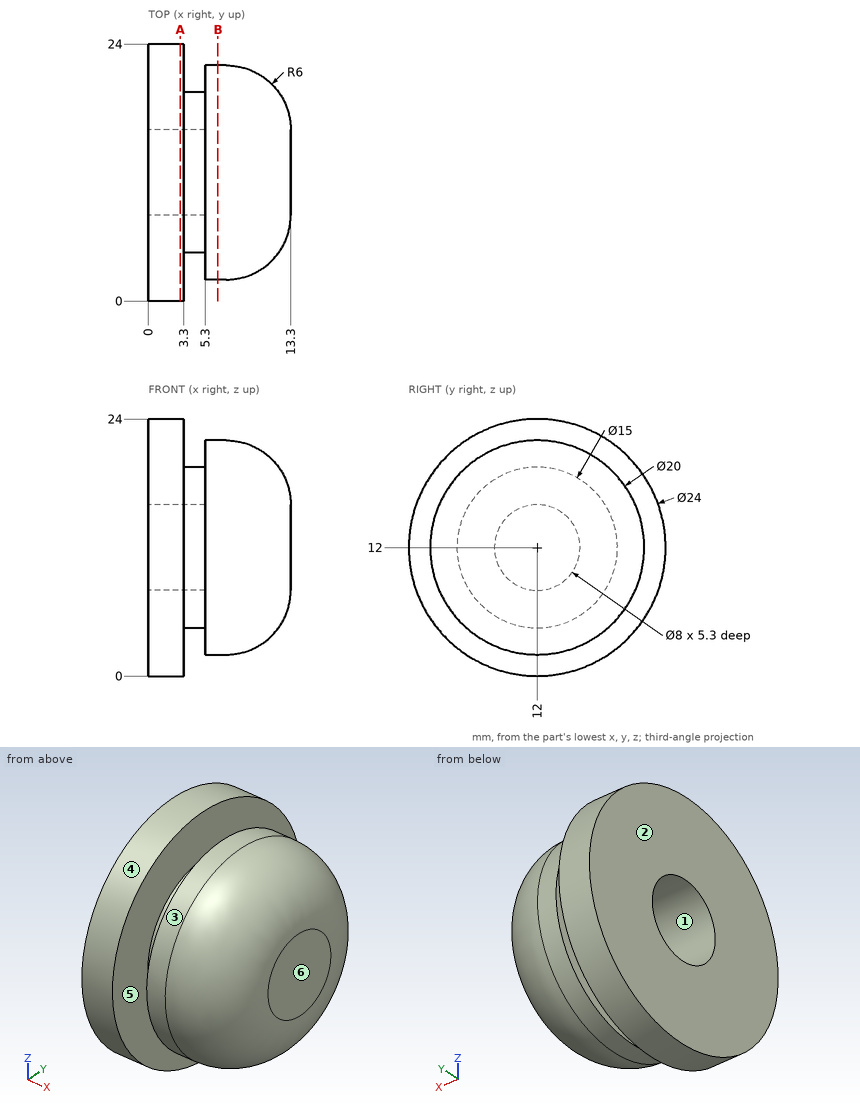
Geometry check sheet. Reference: drawing and pictorial views, mm from the part's lowest x, y, z. A direction names the side the tool comes from. Coordinates: 2 decimals unless noted, no trailing zeros. Loops run counter-clockwise (first coordinate to the right, second up) from the corner with the lowest first, then second, coordinate; pieces in that order, holes last. Notation, with made-up numbers: (20.5, -12.75) -> (46.5, -12.75) arc R24 ccw to (46.5, 25.25) -> close; hole circle Ø4 at (-18, 70.5). An arc over 180 degrees is marked (long way). Put each result on its own line as item: value.
1) Cross-section at B-B on x = 6.5. Record the boundary of the cut face in (y, z), plus the area to 3 significant figures.
Result set:
outline: circle Ø20 at (12, 12)
area: 314 mm^2
2) Tool access check on the marked faces 1, 2 and 3. Record the directions out of +Z, -Z, +X, -X, +Y, -Y that give a thin tool (end or side, any length) a straight path to the whole face; none if there is none.
Result set:
face 1: -X
face 2: +Z, -Z, -X, +Y, -Y
face 3: +X
3) Cross-section at A-A on x = 3. Record the boundary of the cut face in (y, z).
Result set:
outline: circle Ø24 at (12, 12); hole circle Ø8 at (12, 12)
4) Thickness scan on line 1 (Y direction, x = 3.7, z = 12); line 2 (Y direction, x = 3.15, z = 12); line 3 (X direction, y = 14, z = 12). Record the ranges inside material, lowest first.
Result set:
line 1: y = 4.5 to 8, 16 to 19.5
line 2: y = 0 to 8, 16 to 24
line 3: x = 5.3 to 13.3
5) Release check for a two-part mould opening along X. For the marked faces 4, 5 and 6 record: released by +X, released by -X, zero draft, split by the parting line, or undercut.
Result set:
face 4: zero draft
face 5: undercut
face 6: released by +X
6) Gauge pin test, flat ends, axial feed: pin 1 Ø3 at (x, y) = (3.5, 8.5) entering from +Z; pin 2 Ø1 at (x, y) = (10, 15) entering from -Z; pin 3 Ø4 at (y, z) = (5.5, 13.5) entering from +X. Record the tip position at first contact, or that the pin passes through.
Result set:
pin 1: stops at z = 23.83
pin 2: stops at z = 2.85
pin 3: stops at x = 13.26
